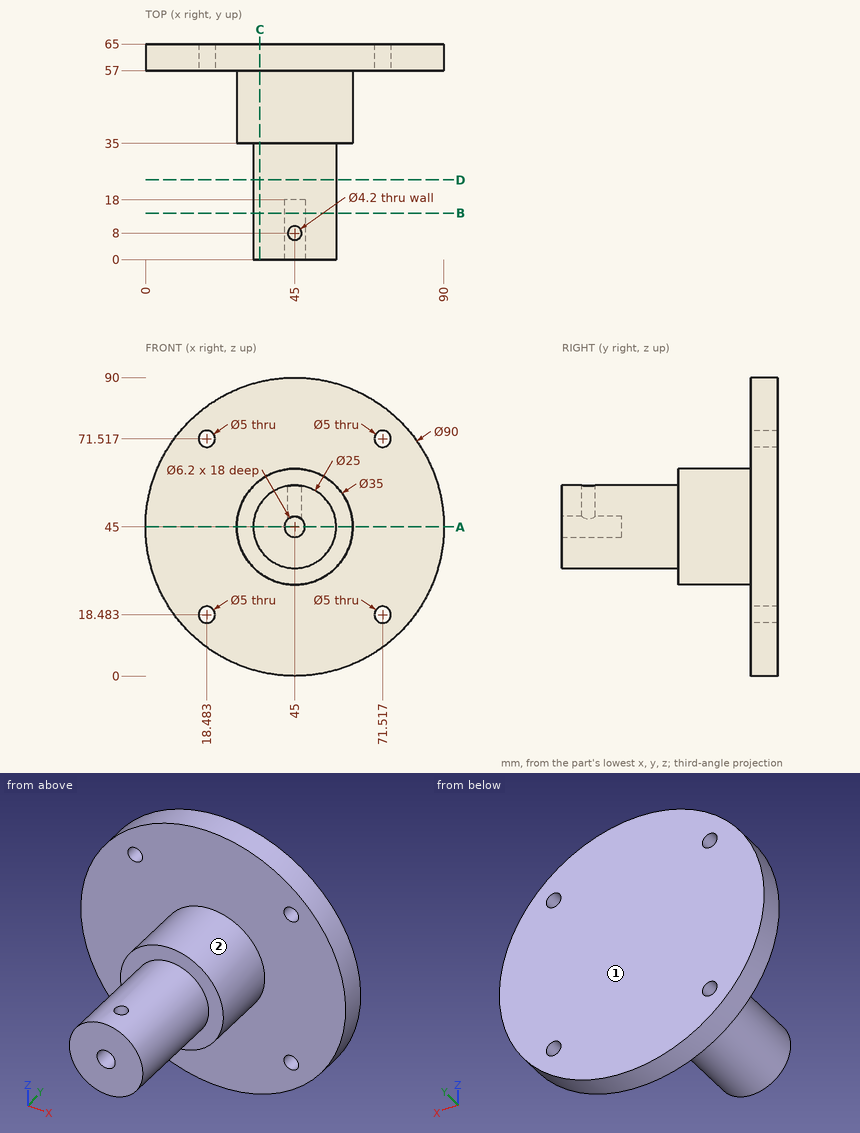
Drawing for the job (mm, zero at the part's lowest x, y, z). A direction names the side the tool comes from. Round coordinates to 2 decimals unless told otherwise and drop trailing zeros. Write each loop counter-clockwise with the first axis right and the second up, starting at its lowest first coordinate (ties: lowest second). Pieces come first, ordered by that corner, then holes. Notation, with made-up numbers: M 73.5,46.25 L 86.5,46.25 A25 cw 86.5,58.25 Z; hole C 42,61 d6. An arc over 180 degrees is marked long. Answer as a JSON object with one key per item and string values. Group by question number.
(1) Cut at C-C (x = 34.5). Give the cut face in (y, z).
(2) Cut at A-A (z = 45). Give the cut face in (x, y), and give its area (3 significant figures).
(3) Drill centre lines: L1, parallel to Y at x = 61, z = 85; L2, parallel to X at y = 7.5, z = 45; L3, parallel to Y at x = 46.5, z = 28.5. Where is each one in solid material? Low to high.
(4) Flat gauge pins, fed straight in: pin 1 (6.5 mm diameter, centred on x = 71.52, z = 18.48, fed in from -Y); pin 2 (3 mm diameter, centred on x = 39.5, y = 7, fed in from +Z); pin 3 (2 mm diameter, centred on y = 36, z = 43, fed in from -X); pin 4 (3 mm diameter, centred on x = 71.52, z = 71.52, fed in from -Y). Where does each tip first touch, or does it go through?
(5) Cut at B-B (y = 14). Give the cut face in (x, z).
(6) Which spindle directions (+Z, -Z, +X, -X, +Y, -Y) get a long thin tool onto all of the face, cutting with end or side? Do the marked faces 1 and 2. Say none if no direction does.
(7) Cut at D-D (y = 24). Give the cut face in (x, z).
Responses:
{
 "1": {"outline": "M 0,38.22 L 35,38.22 L 35,31 L 57,31 L 57,1.24 L 65,1.24 L 65,88.76 L 57,88.76 L 57,59 L 35,59 L 35,51.78 L 0,51.78 Z"},
 "2": {"outline": "M 0,57 L 27.5,57 L 27.5,35 L 32.5,35 L 32.5,0 L 41.9,0 L 41.9,18 L 48.1,18 L 48.1,0 L 57.5,0 L 57.5,35 L 62.5,35 L 62.5,57 L 90,57 L 90,65 L 0,65 Z", "area": "2,250 mm2"},
 "3": {"L1": "y = 57 to 65", "L2": "x = 32.5 to 41.9, 48.1 to 57.5", "L3": "y = 35 to 65"},
 "4": {"pin 1": "stops at y = 57", "pin 2": "stops at z = 56.84", "pin 3": "stops at x = 27.53", "pin 4": "passes through"},
 "5": {"outline": "C 45,45 d25; hole C 45,45 d6.2"},
 "6": {"face 1": "+Z, -Z, +X, -X, +Y", "face 2": "-Y"},
 "7": {"outline": "C 45,45 d25"}
}
